from build123d import *

# Parameters (mm, degrees)
SKETCH_1_W          = 40
SKETCH_1_H          = 6
EXTRUDE_1_DEPTH     = 5
SKETCH_3_R          = 3
EXTRUDE_2_DEPTH     = 5
CUT_EXTRUDE_1_DEPTH = 21.832666656
FILLET_1_RADIUS     = 3
FILLET_1_LENGTH     = 5
SKETCH_5_R          = 1.5
CUT_EXTRUDE_2_DEPTH = 23.561028345
SKETCH_6_R          = 2.5
CUT_EXTRUDE_3_DEPTH = 3
CHAMFER_2_SIZE      = 1
SKETCH_7_R          = 4
EXTRUDE_3_DEPTH     = 10
SKETCH_8_R          = 1.5
CUT_EXTRUDE_4_DEPTH = 24.600847442
SKETCH_9_R          = 3
CUT_EXTRUDE_5_DEPTH = 2
SKETCH_10_R         = 1.6
CUT_EXTRUDE_6_DEPTH = 24.600847442
EXTRUDE_START       = -10
SKETCH_11_R         = 5
SKETCH_11_R_2       = 1.6
EXTRUDE_4_DEPTH     = 10
SKETCH_12_R         = 3
CUT_EXTRUDE_7_DEPTH = 4


with BuildPart() as part:
    # Эскиз1 → Бобышка-Вытянуть1 (new body)
    with BuildSketch(Plane.XY):
        Rectangle(SKETCH_1_W, SKETCH_1_H)
    extrude(amount=EXTRUDE_1_DEPTH)

    # Эскиз3 → Бобышка-Вытянуть2 (add)
    with BuildSketch(Plane(origin=(0, 0, 0), x_dir=(-1, 0, 0), z_dir=(0, 0, -1))):
        with Locations((17, 0)):
            Circle(SKETCH_3_R)
    extrude(amount=EXTRUDE_2_DEPTH)

    # Эскиз4 → Вырез-Вытянуть1 (cut, through all)
    with BuildSketch(Plane(origin=(0, 0, 0), x_dir=(-1, 0, 0), z_dir=(0, 0, -1))):
        with BuildLine():
            Line((20, 3), (17, 3))
            ThreePointArc((17, 3), (19.121320344, 2.121320344), (20, 0))
            Line((20, 0), (20, 3))
        make_face()
        with BuildLine():
            Line((20, -3), (20, 0))
            ThreePointArc((20, 0), (19.121320344, -2.121320344), (17, -3))
            Line((17, -3), (20, -3))
        make_face()
    extrude(amount=-CUT_EXTRUDE_1_DEPTH, mode=Mode.SUBTRACT)

    # Скругление1: full round fillet: the end face becomes a half cylinder, R = half its width
    fillet_1_face = Plane((20, 0, 2.5), x_dir=(0, 0, -1), z_dir=(1, 0, 0))  # on the end face: x along it, z out of the body
    fillet_1_slab = fillet_1_face.offset(-FILLET_1_RADIUS / 2) * Box(FILLET_1_LENGTH, 2 * FILLET_1_RADIUS, FILLET_1_RADIUS, mode=Mode.PRIVATE)  # the body's end, R deep
    fillet_1_round = Plane((17, 0, 2.5), x_dir=(1, 0, 0), z_dir=(0, 0, -1)) * Cylinder(FILLET_1_RADIUS, FILLET_1_LENGTH, mode=Mode.PRIVATE)  # its axis R under the face
    add(fillet_1_slab - fillet_1_round, mode=Mode.SUBTRACT)

    # Эскиз5 → Вырез-Вытянуть2 (cut, through all)
    with BuildSketch(Plane.XY.offset(5)):
        with Locations((-17, 0)):
            Circle(SKETCH_5_R)
        with BuildLine():
            Line((-9, 1.5), (17, 1.5))
            ThreePointArc((17, 1.5), (18.5, 0), (17, -1.5))
            Line((17, -1.5), (-9, -1.5))
            ThreePointArc((-9, -1.5), (-10.5, 0), (-9, 1.5))
        make_face()
    extrude(amount=-CUT_EXTRUDE_2_DEPTH, mode=Mode.SUBTRACT)

    # Эскиз6 → Вырез-Вытянуть3 (cut)
    with BuildSketch(Plane.XY.offset(5)):
        with Locations((-17, 0)):
            Circle(SKETCH_6_R)
    extrude(amount=-CUT_EXTRUDE_3_DEPTH, mode=Mode.SUBTRACT)

    # Фаска2
    chamfer_2_edges = [part.edges().sort_by_distance(p)[0] for p in [
        (4, -1.5, 0),
        (18.5, 0, 0),
        (4, 1.5, 0),
        (-10.5, 0, 0),
        (4, 1.5, 5),
        (-10.5, 0, 5),
        (4, -1.5, 5),
        (18.5, 0, 5),
    ]]
    chamfer(chamfer_2_edges, length=CHAMFER_2_SIZE)

    # Эскиз7 → Бобышка-Вытянуть3 (add)
    with BuildSketch(Plane.XY.offset(5)):
        with Locations((-17, 0)):
            Circle(SKETCH_7_R)
    extrude(amount=-EXTRUDE_3_DEPTH)

    # Эскиз8 → Вырез-Вытянуть4 (cut, through all)
    with BuildSketch(Plane.XY.offset(5)):
        with Locations((-17, 0)):
            Circle(SKETCH_8_R)
    extrude(amount=-CUT_EXTRUDE_4_DEPTH, mode=Mode.SUBTRACT)

    # Эскиз9 → Вырез-Вытянуть5 (cut)
    with BuildSketch(Plane.XY.offset(5)):
        with Locations((-17, 0)):
            Circle(SKETCH_9_R)
    extrude(amount=-CUT_EXTRUDE_5_DEPTH, mode=Mode.SUBTRACT)

    # Эскиз10 → Вырез-Вытянуть6 (cut, through all)
    with BuildSketch(Plane.XY.offset(5)):
        with Locations((-17, 0)):
            Circle(SKETCH_10_R)
    extrude(amount=-CUT_EXTRUDE_6_DEPTH, mode=Mode.SUBTRACT)

    # Эскиз11 → Бобышка-Вытянуть4 (add)
    with BuildSketch(Plane(origin=(0, 0, -5), x_dir=(-1, 0, 0), z_dir=(0, 0, -1)).offset(EXTRUDE_START)):
        with Locations((17, 0)):
            Circle(SKETCH_11_R)
        with Locations(Location((17, 0, 0), (0, 0, 180))):
            Circle(SKETCH_11_R_2, mode=Mode.SUBTRACT)
    extrude(amount=EXTRUDE_4_DEPTH)

    # Эскиз12 → Вырез-Вытянуть7 (cut)
    with BuildSketch(Plane.XY.offset(5)):
        with Locations((-17, 0)):
            Circle(SKETCH_12_R)
    extrude(amount=-CUT_EXTRUDE_7_DEPTH, mode=Mode.SUBTRACT)


solid = part.part
Can you work these out from the model? Positions are in its coordinate system, mm. A direction names the side the tool comes from. Round coordinates to 2 decimals unless told otherwise and drop trailing zeros. Write each loop counter-clockwise with the first axis right and the second up, starting at its lowest first coordinate (ties: lowest second). Pieces come first, ordered by that corner, then holes. Notation, with made-up numbers: M 30,-23 L 73,-23 A25 cw 73,3 Z; hole C -24,81.5 d2. An arc over 180 degrees is marked long. Use a Markdown table: item, result.
Item 1: I want a section at C-C (z = 2.75). List the corners of the cut face in (x, y) for me.
Found:
| item | result |
|---|---|
| outline | M -13,-3 L 17,-3 A3 ccw 17,3 L -13,3 A5 ccw long Z; hole C -17,0 d6; hole M -9,-1.5 L 17,-1.5 A1.5 ccw 17,1.5 L -9,1.5 A1.5 ccw Z |
Item 2: If I drill on line 1 along Y through (x, z) = (10.5, 1.75); line 2 along Y through (x, z) = (-17, 3.65); line 3 along Z through (x, y) = (12, -2.5), over which ranges is the centre line in solid material (lowest first)? Write a range as [from, to].
Found:
| item | result |
|---|---|
| line 1 | y = [-3, -1.5], [1.5, 3] |
| line 2 | y = [-5, -3], [3, 5] |
| line 3 | z = [0, 5] |
Item 3: I want a section at A-A (y = 0). List the corners of the cut face in (x, z) for me, and give its area (3 significant figures).
Found:
| item | result |
|---|---|
| outline | M -22,-5 L -18.6,-5 L -18.6,1 L -20,1 L -20,5 L -22,5 Z; M -15.4,-5 L -12,-5 L -12,0 L -11.5,0 L -10.5,1 L -10.5,4 L -11.5,5 L -14,5 L -14,1 L -15.4,1 Z; M 18.5,1 L 19.5,0 L 20,0 L 20,5 L 19.5,5 L 18.5,4 Z |
| area | 69.8 mm2 |
Item 4: For pin 1 Ø5.5 at (x, z) = (0.5, 3) entering from -Y; pin 2 Ø1 at (x, z) = (1, -1.5) entering from -Y; pin 3 Ø5 at (x, y) = (8.5, 1.5) entering from -Z; pin 4 Ø1.5 at (x, z) = (7, 3) entering from +Y, each with a flat end and sliding along its axis, tell me the tip position at first contact or that it passes through.
Found:
| item | result |
|---|---|
| pin 1 | stops at y = -3 |
| pin 2 | passes through |
| pin 3 | stops at z = 0 |
| pin 4 | stops at y = 3 |
Item 5: I want a section at D-D (x = -17). List the corners of the cut face in (y, z) for me.
Found:
| item | result |
|---|---|
| outline | M -5,-5 L -1.6,-5 L -1.6,1 L -3,1 L -3,5 L -5,5 Z; M 1.6,-5 L 5,-5 L 5,5 L 3,5 L 3,1 L 1.6,1 Z |
Item 6: I want a section at B-B (x = 5). List the corners of the cut face in (y, z) for me, and give its area (3 significant figures).
Found:
| item | result |
|---|---|
| outline | M -3,0 L -2.5,0 L -1.5,1 L -1.5,4 L -2.5,5 L -3,5 Z; M 1.5,1 L 2.5,0 L 3,0 L 3,5 L 2.5,5 L 1.5,4 Z |
| area | 13.0 mm2 |
Item 7: Which directions (+Z, -Z, +X, -X, +Y, -Y) give clear straight access to the entire face, cutting with the end or side of a thin tool? Please do faces 1 (the face through (3.8, 2, 0.5)), 2 (the face through (2, -3, 2)), 3 (the face through (2, 3, 2)), 4 (the face through (18.7, 0, 4.2)), 5 (the face through (-10.5, 0, 2.5)).
Found:
| item | result |
|---|---|
| face 1 | -Z |
| face 2 | +Z, -Z, +X, -Y |
| face 3 | +Z, -Z, +X, +Y |
| face 4 | +Z |
| face 5 | +Z, -Z |
